from build123d import *

# Parameters (mm, degrees)
SKETCH1_R           = 17.5
SKETCH1_R_2         = 4
SKETCH1_R_3         = 0.8
BOSS_EXTRUDE1_DEPTH = 3.65


with BuildPart() as part:
    # Sketch1 → Boss-Extrude1 (new body)
    with BuildSketch(Plane.XY):
        Circle(SKETCH1_R)
        Circle(SKETCH1_R_2, mode=Mode.SUBTRACT)
        with Locations((6.75, 0)):
            Circle(SKETCH1_R_3, mode=Mode.SUBTRACT)
        with Locations((0, 8.75)):
            Circle(SKETCH1_R_3, mode=Mode.SUBTRACT)
        with Locations(Location((0, -8.75, 0), (0, 0, 180))):
            Circle(SKETCH1_R_3, mode=Mode.SUBTRACT)
        with Locations(Location((-6.75, 0, 0), (0, 0, 180))):
            Circle(SKETCH1_R_3, mode=Mode.SUBTRACT)
    extrude(amount=BOSS_EXTRUDE1_DEPTH)


solid = part.part
The listing builds one solid part. Answer for the finished solid, in the listing's coordinates (mm). Coordinates: 2 decimals unless noted, no trailing zeros. Write each loop counter-clockwise with the first axis right and the second up, starting at its lowest first coordinate (ties: lowest second). Pieces come first, ordered by that corner, then holes. Notation, with made-up numbers: (-33.5, 69) -> (16.5, 69) arc R24 ccw to (16.5, 108) -> close; hole circle Ø4 at (60, 10). An arc over 180 degrees is marked (long way). One line per question, with ' | ' between items.
1. Straight lines are drawn through the part: line 1 (Y direction, x = 0, z = 0.75); line 2 (Y direction, x = 6.75, z = 2.45); line 3 (X direction, y = 3, z = 3.2). For each, find the intervals that lie inside material, in ascending order.
Verdict:
line 1: y = -17.5 to -9.55, -7.95 to -4, 4 to 7.95, 9.55 to 17.5 | line 2: y = -16.15 to -0.8, 0.8 to 16.15 | line 3: x = -17.24 to -2.65, 2.65 to 17.24
2. Section C-C (z = 0.55) is taken. Determine the outline of the cut face in (x, y).
Verdict:
outline: circle Ø35 at (0, 0); hole circle Ø1.6 at (-6.75, 0); hole circle Ø8 at (0, 0); hole circle Ø1.6 at (0, -8.75); hole circle Ø1.6 at (0, 8.75); hole circle Ø1.6 at (6.75, 0)
3. Given pin 1 Ø2 at (y, z) = (10, 2) entering from +X, flat-ended and moving along its own axis, determine where the tip first touches the part or whether it passes through.
Verdict:
pin 1: stops at x = 15.01
4. Section D-D (y = -8.75) is taken. Determine the outline of the cut face in (x, z).
Verdict:
outline: (-15.16, 0) -> (-0.8, 0) -> (-0.8, 3.65) -> (-15.16, 3.65) -> close; (0.8, 0) -> (15.16, 0) -> (15.16, 3.65) -> (0.8, 3.65) -> close
5. Section B-B (x = 0) is taken. Determine the outline of the cut face in (y, z).
Verdict:
outline: (-17.5, 0) -> (-9.55, 0) -> (-9.55, 3.65) -> (-17.5, 3.65) -> close; (-7.95, 0) -> (-4, 0) -> (-4, 3.65) -> (-7.95, 3.65) -> close; (4, 0) -> (7.95, 0) -> (7.95, 3.65) -> (4, 3.65) -> close; (9.55, 0) -> (17.5, 0) -> (17.5, 3.65) -> (9.55, 3.65) -> close
6. Section A-A (y = 0) is taken. Determine the outline of the cut face in (x, z), and give its area (3 significant figures).
Verdict:
outline: (-17.5, 0) -> (-7.55, 0) -> (-7.55, 3.65) -> (-17.5, 3.65) -> close; (-5.95, 0) -> (-4, 0) -> (-4, 3.65) -> (-5.95, 3.65) -> close; (4, 0) -> (5.95, 0) -> (5.95, 3.65) -> (4, 3.65) -> close; (7.55, 0) -> (17.5, 0) -> (17.5, 3.65) -> (7.55, 3.65) -> close | area: 86.9 mm^2
7. For a pull along X with two mould halves and no side action, classify faces 1 (the cylindrical face through (-13.887, -10.648, 1.799)), 2 (the flat face through (4, -4, 0)), 3 (the cylindrical face through (5.95, 0.04, 1.8)) as released by +X, released by -X, zero draft, split by the parting line, or undercut.
Verdict:
face 1: split by the parting line | face 2: zero draft | face 3: undercut
